from build123d import *

# Parameters (mm, degrees)
BASEHEAD_DEPTH      = 9.25
BOSS_EXTRUDE1_DEPTH = 11


with BuildPart() as part:
    # Sketch1 → BaseHead (new body)
    with BuildSketch(Plane(origin=(0, 0, 0), x_dir=(0, 0, -1), z_dir=(1, 0, 0))):
        Polygon((10.5, 6.062177826), (10.5, -6.062177826), (0, -12.124355653), (-10.5, -6.062177826), (-10.5, 6.062177826), (0, 12.124355653), align=None)
    extrude(amount=BASEHEAD_DEPTH)

    # BodySke → BaseBody (revolve)
    with BuildSketch(Plane.XY, mode=Mode.PRIVATE) as basebody_sk:
        Polygon((0, 0), (59.25, 0), (59.25, 5.8985), (58.1485, 7), (0, 7), align=None)
    revolve(basebody_sk.sketch.rotate(Axis((0, 0, 0), (1, 0, 0)), 90), axis=Axis((0, 0, 0), (1, 0, 0)))

    # Sketch3 → HeadChamfer (revolve, cut)
    with BuildSketch(Plane.XY):
        Polygon((0, 10.5), (3.824573519, 17.124355653), (3.824573519, 22.124355653), (-10, 22.124355653), (-10, 10.5), align=None)
    revolve(axis=Axis((0, 0, 0), (1, 0, 0)), mode=Mode.SUBTRACT)

    # Sketch4 → Boss-Extrude1 (add)
    with BuildSketch(Plane(origin=(44.25, 0, 0), x_dir=(0, 0, -1), z_dir=(1, 0, 0))):
        Polygon((0, 12.124355653), (-10.5, 6.062177826), (-10.5, -6.062177826), (0, -12.124355653), (10.5, -6.062177826), (10.5, 6.062177826), align=None)
    extrude(amount=BOSS_EXTRUDE1_DEPTH)


solid = part.part
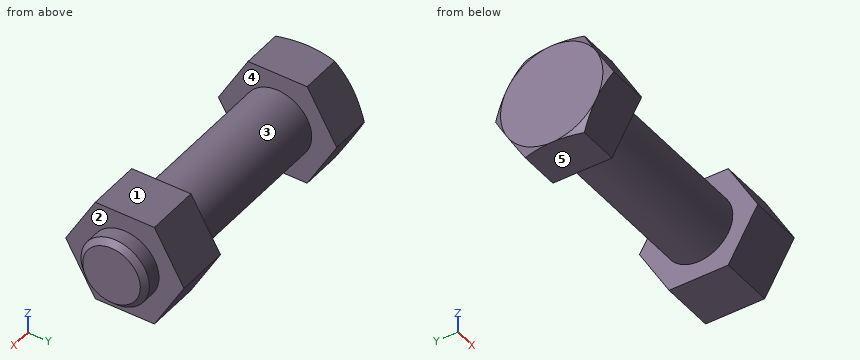
Part model, mm, in its own coordinate system. Face numbers are marked on the shaded views. A direction names the side the tool comes from. Coordinates: 2 decimals unless noted, no trailing zeros. Order: outer loops, then holes, each group sorted by start corner. A loop starts at its lowest first (then second) coordinate and runs counter-clockwise, first axis right, second up.
(1) Tool access for the marked faces 4 and 5: list every direction of +Z, -Z, +X, -X, +Y, -Y with a clear straight run to the whole face (end or side of a thin tool).
Check sheet entries:
face 4: none
face 5: -Z, +X, -X, +Y, -Y
(2) Slice it at A-A, the plane x = 8. Write the cut outline in (y, z), and give its area (3 significant figures).
Check sheet entries:
outline: (-12.12, 0) - (-6.06, -10.5) - (6.06, -10.5) - (12.12, 0) - (6.06, 10.5) - (-6.06, 10.5) - close
area: 382 mm2
(3) Pull direction X, two halves, no side cores. Call the marked faces 1, 2 and 3: pulls with the +X half, pulls with the -X half, needs draft (parallel to the pull), parting line crosses it, or undercut.
Check sheet entries:
face 1: needs draft
face 2: pulls with the +X half
face 3: undercut
(4) Slice it at B-B, the plane x = 38.5. Write the cut outline in (y, z), and give its area (3 significant figures).
Check sheet entries:
outline: circle Ø14 at (0, 0)
area: 154 mm2
(5) Pin check, flat tips, straight feed: pin 1 Ø12 at (x, z) = (31, -5) entering from +Y; pin 2 Ø8 at (x, z) = (33, 6) entering from +Y; pin 3 Ø1.5 at (y, z) = (-9.5, 4) entering from +X. Stop position of each tip, or through.
Check sheet entries:
pin 1: stops at y = 7
pin 2: stops at y = 6.71
pin 3: stops at x = 55.25
(6) Probe L1, parallel to X at y = 7.5, z = -0.25; L2, parallel to Y at x = 20, z = -3.5; L3, parallel to Y at x = 41, z = 3. List the from-to ranges inside material, lowest first.
Check sheet entries:
L1: x = 0 to 9.25, 44.25 to 55.25
L2: y = -6.06 to 6.06
L3: y = -6.32 to 6.32
